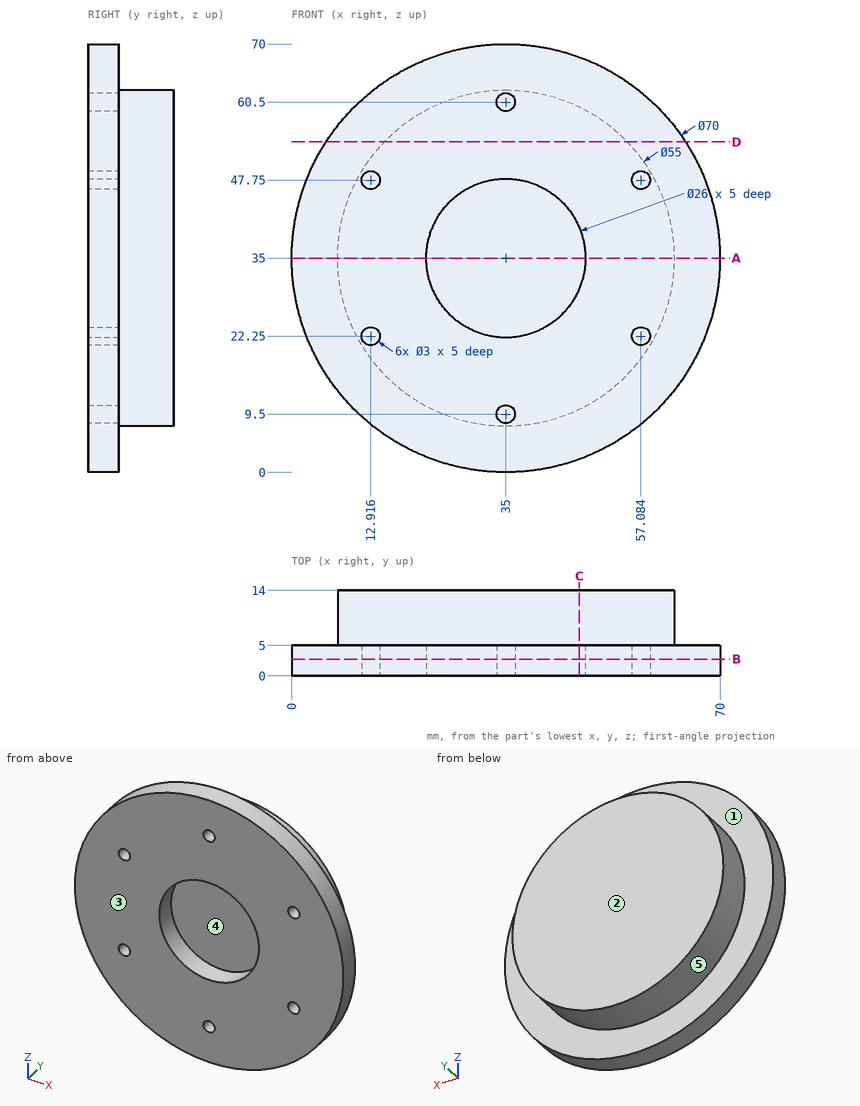
Job drawing, mm, ordinate dimensions from the low corner. One solid piece. A direction names the side the tool comes from. Coordinates: 2 decimals unless noted, no trailing zeros. Loops run counter-clockwise (first coordinate to the right, second up) from the corner with the lowest first, then second, coordinate; pieces in that order, holes last. Notation, with made-up numbers: (-0.75, -22) - (42.25, -22) arc R27 cw to (42.25, 5) - close; hole circle Ø6 at (75.25, 53). An arc over 180 degrees is marked (long way). Answer as a JSON object with one key per item and string values. Group by question number.
(1) Cut at D-D (z = 54). Give the cut face in (x, y), then the cut area to 3 significant figures.
(2) Tool access for the marked faces 1 and 2: list every direction of +Z, -Z, +X, -X, +Y, -Y with a clear straight run to the whole face (end or side of a thin tool).
(3) Probe line 1 along Y through (x, z) = (45.5, 29); line 2 along X through (y, z) = (1.4, 60.5) (1 decimal); line 3 along Z through (x, y) = (24.5, 2.5) (1 decimal). List the from-to ranges inside material, lowest first.
(4) Flat gauge pins, fed straight in: pin 1 (1.5 mm diameter, centred on x = 60, y = 2, fed in from -Z); pin 2 (5 mm diameter, centred on x = 58.5, y = 2, fed in from +Z); pin 3 (3 mm diameter, centred on y = 10, z = 20.5, fed in from -X). Where does each tip first touch, or does it go through?
(5) Two-plate mould, pull along X, no slides. Class the marked faces 3, 4 and 5: released by +X, released by -X, zero draft, split by the parting line, or undercut.
(6) Cut at B-B (y = 2.75). Give the cut face in (x, z), then the cut area to 4 significant figures.
(7) Cut at A-A (z = 35). Give the cut face in (x, y), then the cut area to 3 significant figures.
(8) Cut at C-C (x = 47). Give the cut face in (y, z).
Geometry says:
{
 "1": {"outline": "(5.61, 0) - (64.39, 0) - (64.39, 5) - (54.88, 5) - (54.88, 14) - (15.12, 14) - (15.12, 5) - (5.61, 5) - close", "area": "652 mm^2"},
 "2": {"face 1": "+Y", "face 2": "+Z, -Z, +X, -X, +Y"},
 "3": {"line 1": "y = 5 to 14", "line 2": "x = 11 to 33.5, 36.5 to 59", "line 3": "z = 1.6 to 27.3, 42.7 to 68.4"},
 "4": {"pin 1": "stops at z = 9.76", "pin 2": "stops at z = 63", "pin 3": "stops at x = 10.77"},
 "5": {"face 3": "zero draft", "face 4": "undercut", "face 5": "split by the parting line"},
 "6": {"outline": "circle Ø70 at (35, 35); hole circle Ø3 at (12.92, 22.25); hole circle Ø3 at (12.92, 47.75); hole circle Ø26 at (35, 35); hole circle Ø3 at (35, 9.5); hole circle Ø3 at (35, 60.5); hole circle Ø3 at (57.08, 22.25); hole circle Ø3 at (57.08, 47.75)", "area": "3,275 mm^2"},
 "7": {"outline": "(0, 0) - (22, 0) - (22, 5) - (48, 5) - (48, 0) - (70, 0) - (70, 5) - (62.5, 5) - (62.5, 14) - (7.5, 14) - (7.5, 5) - (0, 5) - close", "area": "715 mm^2"},
 "8": {"outline": "(0, 2.12) - (5, 2.12) - (5, 10.26) - (14, 10.26) - (14, 59.74) - (5, 59.74) - (5, 67.88) - (0, 67.88) - (0, 40) - (5, 40) - (5, 30) - (0, 30) - close"}
}
